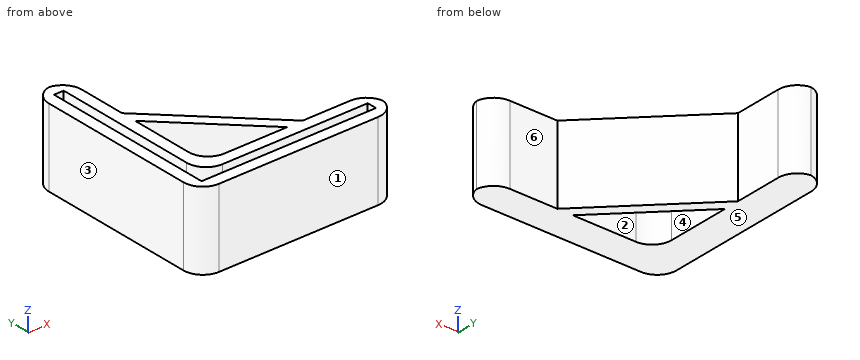
```python
from build123d import *

# Parameters (mm, degrees)
F1_DEPTH    = 20
F2_DEPTH    = 6
F3_T1_DEPTH = 20
F3_T3_DEPTH = 45
F4_R        = 5


# Not quite as in the source:
# - a fillet or chamfer that OpenCascade refuses, or shapes differently, is made with other operations: its cross-section is extruded or revolved along the edge and cut away or added


with BuildPart() as f1:
    # F0 (on Top) → F1 (new body)
    with BuildSketch(Plane.XY):
        Polygon((5.5, 30.75), (5.5, 48), (-3, 48), (-3, -3), (48, -3), (48, 5.5), (30.75, 5.5), (26.75, 5.5), (5.5, 5.5), (5.5, 26.75), align=None)
        Polygon((0, 0), (0, 45), (2.5, 45), (2.5, 2.5), (45, 2.5), (45, 0), align=None, mode=Mode.SUBTRACT)
        Polygon((30.75, 5.5), (5.5, 30.75), (5.5, 26.75), (26.75, 5.5), align=None)
    extrude(amount=F1_DEPTH)

    # F0 (on Top) → F2 (join)
    with BuildSketch(Plane.XY):
        Polygon((2.5, 45), (0, 45), (0, 0), (45, 0), (45, 2.5), (2.5, 2.5), align=None)
    extrude(amount=F2_DEPTH)

    # F3: fillet of radius 5 on 6 edges, made by hand

    # F3_s2 → F3_t1 (join)
    with BuildSketch(Plane.XY):
        with BuildLine():
            ThreePointArc((10.5, 5.5), (6.9644660941, 6.9644660941), (5.5, 10.5))
            Line((5.5, 10.5), (5.5, 5.5))
            Line((5.5, 5.5), (10.5, 5.5))
        make_face()
    extrude(amount=F3_T1_DEPTH)

    # F3_s4 → F3_t3 (cut)
    with BuildSketch(Plane.XY.offset(-12.5)):
        with BuildLine():
            ThreePointArc((43, 5.5), (46.5355339059, 4.0355339059), (48, 0.5))
            Line((48, 0.5), (48, 5.5))
            Line((48, 5.5), (43, 5.5))
        make_face()
        with BuildLine():
            ThreePointArc((43, -3), (46.5355339059, -1.5355339059), (48, 2))
            Line((48, 2), (48, -3))
            Line((48, -3), (43, -3))
        make_face()
        with BuildLine():
            ThreePointArc((5.5, 43), (4.0355339059, 46.5355339059), (0.5, 48))
            Line((0.5, 48), (5.5, 48))
            Line((5.5, 48), (5.5, 43))
        make_face()
        with BuildLine():
            ThreePointArc((2, 48), (-1.5355339059, 46.5355339059), (-3, 43))
            Line((-3, 43), (-3, 48))
            Line((-3, 48), (2, 48))
        make_face()
        with BuildLine():
            ThreePointArc((-3, 2), (-1.5355339059, -1.5355339059), (2, -3))
            Line((2, -3), (-3, -3))
            Line((-3, -3), (-3, 2))
        make_face()
    extrude(amount=F3_T3_DEPTH, mode=Mode.SUBTRACT)

    # F4
    f4_edges = [f1.edges().sort_by_distance(p)[0] for p in [
        (2.5, 2.5, 13),
    ]]
    fillet(f4_edges, radius=F4_R)


solid = f1.part
```
The listing builds one solid part. Answer for the finished solid, in the listing's coordinates (mm). Face numbers are marked on the shaded views. A direction names the side the tool comes from. Round coordinates to 2 decimals unless told otherwise and drop trailing zeros. Write each loop counter-clockwise with the first axis right and the second up, starting at its lowest first coordinate (ties: lowest second). Pieces come first, ordered by that corner, then holes. Notation, with made-up numbers: (34.25, 69.5) -> (58.25, 69.5) arc R26 ccw to (58.25, 92.5) -> close; hole circle Ø8 at (32, 3). An arc over 180 degrees is marked (long way). Write item = value, one per line.
1) Section A-A on x = 13 is taken. Write down the section's boundary in (y, z).
Check values:
outline = (-3, 0) -> (5.5, 0) -> (5.5, 20) -> (2.5, 20) -> (2.5, 6) -> (0, 6) -> (0, 20) -> (-3, 20) -> close; (19.25, 0) -> (23.25, 0) -> (23.25, 20) -> (19.25, 20) -> close
2) Which of the six approach directions +Z, -Z, +X, -X, +Y, -Y give full straight-line access (tool end or side, diameter ignored) to the marked faces 4, 5 and 6?
Check values:
face_4 = +Z, -Z
face_5 = -Z, +X, -X, +Y, -Y
face_6 = +Z, -Z, +X, +Y
3) Section B-B on z = 12.25 is taken. Write down the section's boundary in (x, y), plus the area to 3 significant figures.
Check values:
outline = (-3, 2) arc R5 ccw to (2, -3) -> (43, -3) arc R5 ccw to (47.94, 1.25) arc R5 ccw to (43, 5.5) -> (30.75, 5.5) -> (5.5, 30.75) -> (5.5, 43) arc R5 ccw to (1.25, 47.94) arc R5 ccw to (-3, 43) -> close; hole (0, 0) -> (45, 0) -> (45, 2.5) -> (7.5, 2.5) arc R5 cw to (2.5, 7.5) -> (2.5, 45) -> (0, 45) -> close; hole (5.5, 10.5) arc R5 ccw to (10.5, 5.5) -> (26.75, 5.5) -> (5.5, 26.75) -> close
area = 642 mm²
4) Section C-C on x = 34 is taken. Write down the section's boundary in (y, z).
Check values:
outline = (-3, 0) -> (5.5, 0) -> (5.5, 20) -> (2.5, 20) -> (2.5, 6) -> (0, 6) -> (0, 20) -> (-3, 20) -> close
5) Section D-D on y = 4.5 is taken. Write down the section's boundary in (x, z).
Check values:
outline = (-3, 0) -> (46, 0) -> (46, 20) -> (3.5, 20) -> (3.5, 6) -> (0, 6) -> (0, 20) -> (-3, 20) -> close
6) Straight lines are drawn through the part: line 1 along X through (y, z) = (21, 9); line 2 along Y through (x, z) = (41.5, 10.5); line 3 along X through (y, z) = (17.5, 13.75). For each, find the intervals that lie inside material, in ascending order. Write a range as [from, to].
Check values:
line_1 = [-3, 0], [2.5, 5.5], [11.25, 15.25]
line_2 = [-3, 0], [2.5, 5.5]
line_3 = [-3, 0], [2.5, 5.5], [14.75, 18.75]
7) For a pull along X with two mould halves and no side action, classify the marked faces 1, 2 and 3 as released by +X, released by -X, zero draft, split by the parting line, or undercut.
Check values:
face_1 = zero draft
face_2 = undercut
face_3 = released by -X
8) Given pin 1 (8 mm diameter, centred on y = 16.5, z = 9, fed in from +X); pin 2 (11 mm diameter, centred on y = 25.5, z = 12, fed in from +X); pin 3 (10 mm diameter, centred on y = 36.5, z = 6.5, fed in from +X), each flat-ended and moving along its own axis, determine where each tip first touches the part or whether it passes through.
Check values:
pin_1 = 23.75
pin_2 = 16.25
pin_3 = 5.5
